Design review of the part shown in the three views and the two pictorial views. Dimensions are in mm from the part's minimum x, y and z. A direction names the side the tool comes from. Coordinates: 2 decimals unless noted, no trailing zeros. Write each loop counter-clockwise with the first axis right and the second up, starting at its lowest first coordinate (ties: lowest second). Pieces come first, ordered by that corner, then holes. Notation, with made-up numbers: (36, 33) -> (90, 33) arc R13 cw to (90, 51) -> close; hole circle Ø8 at (49, 17). An arc over 180 degrees is marked (long way). Answer in a Markdown table with one row per item. Add a question column.
Item 1: Take a section at C-C, the plane z = 2.4. Give the number of separate pieces and of enclosed holes in the cut face, and give its area (3 significant figures).
Item 2: Take a section at B-B, the plane y = 3. Write out the cut boundary in (x, z), and give its area (3 significant figures).
Item 3: Clearance check with flat-ended pins moving along their axes: P1, Ø0.8, axis at y = 1, z = 2.5, coming from the -X side; P2, Ø1.2, axis at x = 19, z = 2, coming from the -Y side. State where each tip first meets the part, or that it passes through.
Item 4: Take a section at D-D, the plane y = 10.5. Write out the cut boundary in (x, z).
Item 5: For the marked faces 1 and 2, list the 3-axis set-ups (+Z, -Z, +X, -X, +Y, -Y) from which the entire face can be reached by the end or side of a thin tool; tool diameter is ignored.
Item 6: To check wall thickness, follow line 1 (X direction, y = 2, z = 3.3); line 2 (Y direction, x = 19.5, z = 2.6); line 3 (Y direction, x = 17.5, z = 4.55). State the ranges of each line that lie inside material, in increasing order.
Item 7: Take a section at A-A, the plane x = 12. Write out the cut boundary in (y, z).
Item 8: Draft analysis for pull direction X (two halves, no side actions). For the marked faces 3, 4 and 5, state which applies: released by +X, released by -X, zero draft, split by the parting line, or undercut.
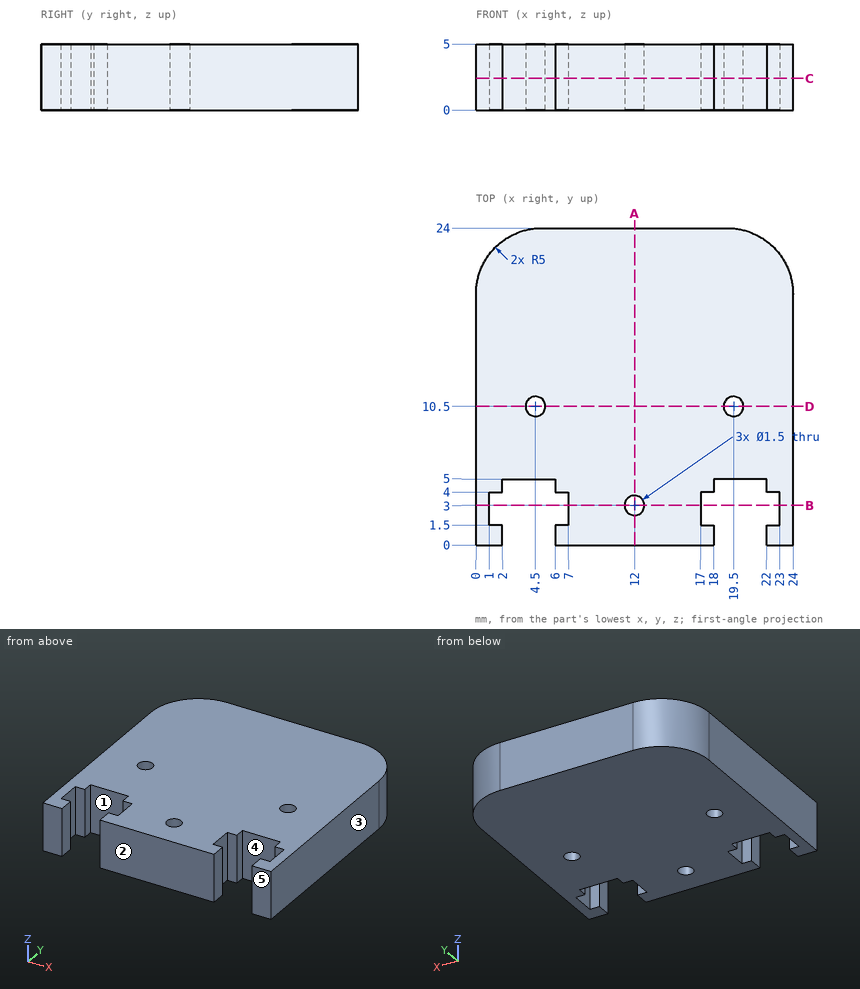
Answers:
| question | item | result |
|---|---|---|
| 1 | separate pieces | 1 |
| 1 | enclosed holes | 3 |
| 1 | area | 510 mm^2 |
| 2 | outline | (0, 0) -> (1, 0) -> (1, 5) -> (0, 5) -> close; (7, 0) -> (11.25, 0) -> (11.25, 5) -> (7, 5) -> close; (12.75, 0) -> (17, 0) -> (17, 5) -> (12.75, 5) -> close; (23, 0) -> (24, 0) -> (24, 5) -> (23, 5) -> close |
| 2 | area | 52.5 mm^2 |
| 3 | P1 | stops at x = 0 |
| 3 | P2 | stops at y = 5 |
| 4 | outline | (0, 0) -> (3.75, 0) -> (3.75, 5) -> (0, 5) -> close; (5.25, 0) -> (18.75, 0) -> (18.75, 5) -> (5.25, 5) -> close; (20.25, 0) -> (24, 0) -> (24, 5) -> (20.25, 5) -> close |
| 5 | face 1 | +Z, -Z, -Y |
| 5 | face 2 | +Z, -Z, +X, -X, -Y |
| 6 | line 1 | x = 0 to 1, 7 to 17, 23 to 24 |
| 6 | line 2 | y = 5 to 9.75, 11.25 to 23.97 |
| 6 | line 3 | y = 0 to 1.5, 4 to 24 |
| 7 | outline | (0, 0) -> (2.25, 0) -> (2.25, 5) -> (0, 5) -> close; (3.75, 0) -> (24, 0) -> (24, 5) -> (3.75, 5) -> close |
| 8 | face 3 | released by +X |
| 8 | face 4 | undercut |
| 8 | face 5 | zero draft |
